```python
from build123d import *

# Parameters (mm, degrees)
BASE_FLANGE1_DEPTH = 12
SKETCH6_R          = 1.5
CUT_EXTRUDE1_DEPTH = 0.7
SKETCH7_R          = 2.15
CUT_EXTRUDE2_DEPTH = 0.7


# Sheet-metal steps are written as plain solids
with BuildPart() as part:
    # Sketch1 → Base-Flange1 (new body)
    with BuildSketch(Plane.XY):
        with BuildLine():
            Line((0, 0), (23.6, 0))
            ThreePointArc((23.6, 0), (24.589949494, 0.410050506), (25, 1.4))
            Line((25, 1.4), (25, 20))
            Line((25, 20), (24.3, 20))
            Line((24.3, 20), (24.3, 1.4))
            ThreePointArc((24.3, 1.4), (24.094974747, 0.905025253), (23.6, 0.7))
            Line((23.6, 0.7), (0, 0.7))
            Line((0, 0.7), (0, 0))
        make_face()
    extrude(amount=BASE_FLANGE1_DEPTH)

    # Sketch6 → Cut-Extrude1 (cut)
    with BuildSketch(Plane(origin=(0, 0.7, 0), x_dir=(1, 0, 0), z_dir=(0, 1, 0))):
        with Locations(Location((7.5, -8, 0), (0, 0, 270))):
            Circle(SKETCH6_R)
        with Locations(Location((17.5, -8, 0), (0, 0, 270))):
            Circle(SKETCH6_R)
        with Locations(Location((11.8, -3.5, 0), (0, 0, 270))):
            Circle(SKETCH6_R)
    extrude(amount=-CUT_EXTRUDE1_DEPTH, mode=Mode.SUBTRACT)

    # Sketch7 → Cut-Extrude2 (cut)
    with BuildSketch(Plane(origin=(25, 0, 0), x_dir=(0, 0, -1), z_dir=(1, 0, 0))):
        with Locations((-8, 15)):
            Circle(SKETCH7_R)
        with Locations((-8, 5)):
            Circle(SKETCH7_R)
    extrude(amount=-CUT_EXTRUDE2_DEPTH, mode=Mode.SUBTRACT)


solid = part.part
```
Build history of the part. All positions in model axes, mm. A direction names the side the tool comes from. Coordinates: 2 decimals unless noted, no trailing zeros. Write each loop counter-clockwise with the first axis right and the second up, starting at its lowest first coordinate (ties: lowest second). Pieces come first, ordered by that corner, then holes.
1. Pull direction Z, two halves, no side cores. Call faces 1 (the flat face through (12, 0.7, 6)), 2 (the cylindrical face through (24.65, 13.09, 7.01)), 3 (the cylindrical face through (24.65, 6.81, 6.84)), 4 (the flat face through (18, 0.4, 12)): released by +Z, released by -Z, zero draft, split by the parting line, or undercut.
Answer block:
face 1: zero draft
face 2: undercut
face 3: undercut
face 4: released by +Z
2. Band-saw the part on A-A, the plane z = 8. Give the cut face in (x, y), and give its area (3 significant figures).
Answer block:
outline: (0, 0) - (6, 0) - (6, 0.7) - (0, 0.7) - close; (9, 0) - (16, 0) - (16, 0.7) - (9, 0.7) - close; (19, 0) - (23.6, 0) arc R1.4 ccw to (25, 1.4) - (25, 2.85) - (24.3, 2.85) - (24.3, 1.4) arc R0.7 cw to (23.6, 0.7) - (19, 0.7) - close; (24.3, 7.15) - (25, 7.15) - (25, 12.85) - (24.3, 12.85) - close; (24.3, 17.15) - (25, 17.15) - (25, 20) - (24.3, 20) - close
area: 20.5 mm2
3. Drop flat-ended pins along their axis: pin 1 (1.5 mm diameter, centred on y = 16.5, z = 4, fed in from -X); pin 2 (1.8 mm diameter, centred on x = 7.5, z = 8, fed in from +Y) (3 decimals); pin 3 (1 mm diameter, centred on x = 15.5, z = 7.5, fed in from +Y). Give the stop position or say it passes through.
Answer block:
pin 1: stops at x = 24.3
pin 2: passes through
pin 3: stops at y = 0.7
4. Band-saw the part on B-B, the plane x = 7.5. Give the cut face in (y, z), and give its area (3 significant figures).
Answer block:
outline: (0, 0) - (0.7, 0) - (0.7, 6.5) - (0, 6.5) - close; (0, 9.5) - (0.7, 9.5) - (0.7, 12) - (0, 12) - close
area: 6.30 mm2
5. 3-axis set-ups, long thin cutter, end or side, ignore diameter. For faces 5 (the flat face through (12, 0, 6)), 6 (the flat face through (24.3, 11, 6)): which of +Z, -Z, +X, -X, +Y, -Y reach the whole face in a straight line?
Answer block:
face 5: +Z, -Z, +X, -X, -Y
face 6: +Z, -Z, -X, +Y
6. Drill centre lines: probe 1 along Y at (x, z) = (24.8, 8); probe 2 along X at (y, z) = (0.4, 8); probe 3 along Y at (x, z) = (21.5, 1.5). Where is each one in solid material? Low to high.
Answer block:
probe 1: y = 0.68 to 2.85, 7.15 to 12.85, 17.15 to 20
probe 2: x = 0 to 6, 9 to 16, 19 to 24.58
probe 3: y = 0 to 0.7
7. Band-saw the part on D-D, the plane y = 12.5. Give the cut face in (x, z).
Answer block:
outline: (24.3, 0) - (25, 0) - (25, 12) - (24.3, 12) - close
8. Band-saw the part on C-C, the plane y = 5. Give the cut face in (x, z), and give its area (3 significant figures).
Answer block:
outline: (24.3, 0) - (25, 0) - (25, 5.85) - (24.3, 5.85) - close; (24.3, 10.15) - (25, 10.15) - (25, 12) - (24.3, 12) - close
area: 5.39 mm2
